Read the model definition and answer for the solid it produces. Units are mm, in the model's axes. A direction names the side the tool comes from. Coordinates: 2 decimals unless noted, no trailing zeros. Write each loop counter-clockwise with the first axis right and the second up, starting at its lowest first coordinate (ties: lowest second). Pieces come first, ordered by that corner, then holes. Notation, with made-up numbers: (15.25, -9) - (52.25, -9) arc R22 cw to (52.25, 10) - close; hole circle Ø1 at (65.25, 58.5). An arc over 180 degrees is marked (long way). Use a Markdown table: item, result.
Autodesk Inventor part; units mm, degrees
ref_plane "YZ Plane" through (0, 0, 0) normal (1, 0, 0) x (0, 1, 0)
ref_plane "XZ Plane" through (0, 0, 0) normal (0, 1, 0) x (-1, 0, 0)
ref_plane "XY Plane" through (0, 0, 0) normal (0, 0, 1) x (1, 0, 0)
sketch "Sketch2" plane through (0, 0, 0) normal (0, 1, 0) x (-1, 0, 0)
  line L0 (-5.5536, -11.7431) -> (5.5568, -15.0764)
  line L1 (5.5568, -25.2431) -> (-23.9154, -25.2431)
  line L2 (-23.9154, -25.2431) -> (-23.9154, -11.7431)
  line L3 (-5.5536, -11.7431) -> (-23.9154, -11.7431)
  line L4 (5.5568, -25.2431) -> (5.5568, -15.0764)
  circle A0 centre (-23.9154, -18.4931) radius 6.75
  circle A1 centre (-23.9154, -18.4931) radius 2.2
  circle A2 centre (-23.9154, -18.4931) radius 6.202
  circle A3 centre (-24.9154, -18.9931) radius 6.25
  line L5 (-18.8553, -31.0955) -> (-18.419, -3.4058)
  point P0 (0, 0)
  point P1 (0, 0)
  point P2 (-19.4912, -10.8803)
  point P3 (-19.4912, -24.3803)
  point P4 (-23.9154, -12.2912)
  point P5 (-23.9154, -24.6951)
  dimension "d1" = 13.5
  dimension "d0" = 4.4
  dimension "d6" = 0.5
  dimension "d7" = 1
  dimension "d8" = 12.5
extrude "Extrusion1" add sketch "Sketch2" along normal blind 3.85 contours L0 L4 L1 L5 A0 L3 | L5 A0 L3 | A0 L5 A2 L2 | L2 A2 A3 A0 | A0 L5 A2 | L1 A0 L5 | A2 L5 A3 L2 | L2 A3 A2 | A3 A2 L2 A0 | L5 A2 A3 | A2 L5 | A0 A3 L2 | L2 A3 A2 L5 A0 | A3 A2 L2 A1 | L2 A1 A2 A3 | L2 A2 A3
extrude "Extrusion2" add sketch "Sketch2" along normal blind 8.85 contours L0 L4 L1 L5 A0 L3 | L5 A0 L3 | A0 L5 A2 L2 | A0 L5 A2 | L1 A0 L5 | L2 A3 A2 L5 A0 | L2 A2 A3 picked at (-23.6214, -24.9369)
sketch "Sketch3" plane through (0, 8.85, 0) normal (0, 1, 0) x (1, 0, 0)
  line L0 (-5.5568, 25.2431) -> (-5.5568, 15.0764)
  line L1 (-5.5568, 15.0764) -> (5.5536, 11.7431)
  line L2 (5.5536, 11.7431) -> (23.9154, 11.7431)
  line L3 (23.9154, 11.7431) -> (23.9154, 12.2912)
  arc A0 (23.9154, 24.6951) -> (23.9154, 12.2912) centre (23.9154, 18.4931) ccw
  line L4 (23.9154, 24.6951) -> (23.9154, 25.2431)
  line L5 (23.9154, 25.2431) -> (-5.5568, 25.2431)
  line L6 (18.8553, 31.0955) -> (18.419, 3.4058)
  point P0 (0, 0)
  point P1 (18.6062, 15.2873)
  point P2 (18.5504, 11.7431)
  point P3 (18.7631, 25.2431)
  point P4 (18.7099, 21.8646)
extrude "Extrusion3" cut sketch "Sketch3" against normal up to surface (5 mm away) contours L5 L4 A0 L6 | L6 A0 L3 L2
sketch "Sketch4" plane through (-5.5568, 0, -25.2431) normal (-1, 0, 0) x (0, 0, 1)
  line L0 (0, 0) -> (10.1667, 0)
  line L1 (10.1667, 0) -> (10.1667, 8.85)
  line L2 (0, 8.85) -> (10.1667, 8.85)
  line L3 (0, 0) -> (0, 8.85)
  line L4 (9.1667, 7.85) -> (9.1667, 1)
  line L5 (9.1667, 1) -> (1, 1)
  line L6 (1, 1) -> (1, 7.85)
  line L7 (1, 7.85) -> (9.1667, 7.85)
  point P0 (25.2431, 0)
  dimension "d11" = 1
extrude "Extrusion4" cut sketch "Sketch4" against normal blind 8 contours L4 L5 L6 L7
sketch "Sketch5" plane through (-5.5568, 1, -16.0764) normal (0, 1, 0) x (1, 0, 0)
  line L0 (0, 0) -> (0, 8.1667)
  line L1 (0, 0) -> (8, 0)
  line L2 (8, 0) -> (8, 8.1667)
  line L3 (0, 8.1667) -> (8, 8.1667)
  line L4 (8, 4.0834) -> (2.9855, 4.0834) construction
  line L5 (4, 0) -> (4, 4.0834) construction
  circle A0 centre (4, 4.0834) radius 2.55
  point P0 (5.5568, -16.0764)
  dimension "d14" = 5.1
extrude "Extrusion5" add sketch "Sketch5" along normal up to surface (6.85 mm away) contours A0
sketch "Sketch6" plane through (5.5536, 0, -11.7431) normal (0, 0, 1) x (1, 0, 0)
  line L0 (-11.1104, 7.85) -> (-11.1104, 1)
  line L1 (-11.1104, 7.85) -> (-4.8007, 7.85)
  line L2 (-4.8007, 7.85) -> (-4.8007, 1)
  line L3 (-11.1104, 1) -> (-4.8007, 1)
  point P0 (-5.5536, 0)
extrude "Extrusion6" cut sketch "Sketch6" against normal up to surface (4.3333 mm away)
sketch "Sketch7" plane through (-5.5568, 1, -24.2431) normal (0, 0, 1) x (1, 0, 0)
  line L0 (0, 0) -> (0, 6.85)
  line L1 (0, 0) -> (8, 0)
  line L2 (8, 0) -> (8, 6.85)
  line L3 (0, 6.85) -> (8, 6.85)
  point P0 (5.5568, -1)
extrude "Extrusion7" cut sketch "Sketch7" against normal blind 10.25
sketch "Sketch8" plane through (0, 8.85, 0) normal (0, 1, 0) x (1, 0, 0)
  circle A0 centre (-1.5568, 20.1598) radius 2.55
  circle A1 centre (-1.5568, 20.1598) radius 2.55
  line L0 (-5.5568, 25.2431) -> (2.4432, 25.2431)
  point P0 (0, 0)
fillet "Fillet1" radius 3 2 edges at (-5.5568, 8.35, -15.0764) (-5.5568, 0.5, -15.0764)
chamfer "Chamfer1" distance 2 angle 45 2 edges at (-5.5568, 8.35, -25.2431) (-5.5568, 0.5, -25.2431)
chamfer "Chamfer2" distance 2 angle 45 1 edges at (18.7631, 6.35, -25.2431)
fillet "Fillet2" radius 3 1 edges at (18.5504, 6.35, -11.7431)
chamfer "Chamfer3" distance 1 angle 45 7 edges at (6.6031, 8.85, -25.2431) (10.5754, 8.85, -11.7431) (17.7018, 8.85, -12.6052) (18.6016, 8.85, -14.9916) (14.7345, 0, -11.7431) (30.6654, 0, -18.4931) (10.1793, 0, -25.2431)
properties part number "Upper Leg"
(1) For faces 1 (the flat face through (17.76, 6.38, -24.23)), 2 (the flat face through (0.753, 4, -15)), 3 (the flat face through (0.2, 1, -17.8)), determine the directions among +Z, -Z, +X, -X, +Y, -Y from which every point of the face is accessible in a straight line to the end or side of a thin tool.
Report:
| item | result |
|---|---|
| face 1 | -Z, +X, +Y |
| face 2 | +Z, -X |
| face 3 | none |
(2) A cutting plane is placed at A-A, the plane y = 3. Write down the section's boundary in (x, z), and give its area (3 significant figures).
Report:
| item | result |
|---|---|
| outline | circle Ø5.1 at (-1.56, -20.16); (0.75, -16.08) - (2.44, -16.08) - (2.44, -25.24) - (23.92, -25.24) arc R6.75 ccw to (23.92, -11.74) - (5.55, -11.74) - (0.75, -13.18) - close; hole circle Ø4.4 at (23.92, -18.49) |
| area | 371 mm² |
(3) The mould has two halves that part along Y. Classify faces 4 (the flat face through (2.443, 4, -21)), 5 (the cylindrical face through (-4.95, 8.34, -15.5)), 6 (the flat face through (6.439, 8.343, -24.75)): pulls with the +Y half, pulls with the -Y half, needs draft (parallel to the pull), parting line crosses it, or undercut.
Report:
| item | result |
|---|---|
| face 4 | undercut |
| face 5 | needs draft |
| face 6 | pulls with the +Y half |
(4) A cutting plane is placed at C-C, the plane y = 6. Write down the section's boundary in (x, z).
Report:
| item | result |
|---|---|
| outline | circle Ø5.1 at (-1.56, -20.16); (0.75, -16.08) - (2.44, -16.08) - (2.44, -25.24) - (16.76, -25.24) - (18.73, -23.24) - (18.71, -21.86) arc R6.2 cw to (18.61, -15.29) - (18.6, -14.7) arc R3 ccw to (15.6, -11.74) - (5.55, -11.74) - (0.75, -13.18) - close |
(5) A cutting plane is placed at B-B, the plane x = 11.5. Write down the section's boundary in (y, z), and give its area (3 significant figures).
Report:
| item | result |
|---|---|
| outline | (0, -24.24) - (1, -25.24) - (7.85, -25.24) - (8.85, -24.24) - (8.85, -12.74) - (7.85, -11.74) - (1, -11.74) - (0, -12.74) - close |
| area | 117 mm² |
(6) Straight lines are drawn through the part: L1, parallel to Y at x = 25, z = -14; L2, parallel to Z at x = 25, y = 2; L3, parallel to X at y = 7.75, z = -18.5. For each, find the intervals that lie inside material, in ascending order.
Report:
| item | result |
|---|---|
| L1 | y = 0 to 3.85 |
| L2 | z = -25.16 to -20.41, -16.58 to -11.83 |
| L3 | x = -3.49 to 0.38, 2.44 to 17.71 |
(7) A cutting plane is placed at D-D, the plane z = -19.5. Count the separate pieces of the cut face and the enclosed holes in it, and give its area (3 significant figures).
Report:
| item | result |
|---|---|
| separate pieces | 2 |
| enclosed holes | 1 |
| area | 219 mm² |
(8) Each of these flat-tipped pins is pushed along its axis until it touches: P1, Ø1.4, axis at y = 3.5, z = -15, coming from the -X side; P2, Ø0.5, axis at x = 2, y = 2.5, coming from the -Z side; P3, Ø4, axis at x = 20, z = -16.5, coming from the +Y side; P4, Ø2.5, axis at x = 23.92, z = -18.49, coming from the +Y side. Where does it stop, or does it pass through?
Report:
| item | result |
|---|---|
| P1 | stops at x = 0.75 |
| P2 | stops at z = -16.08 |
| P3 | stops at y = 8.48 |
| P4 | passes through |
